Answer from the drawing. Dimensions are ordinates in mm from the lowest x, y and z of the part. Round coordinates to 2 decimals unless told otherwise and drop trailing zeros. Order: outer loops, then holes, each group sorted by start corner. A loop starts at its lowest first (then second) coordinate and runs counter-clockwise, first axis right, second up.
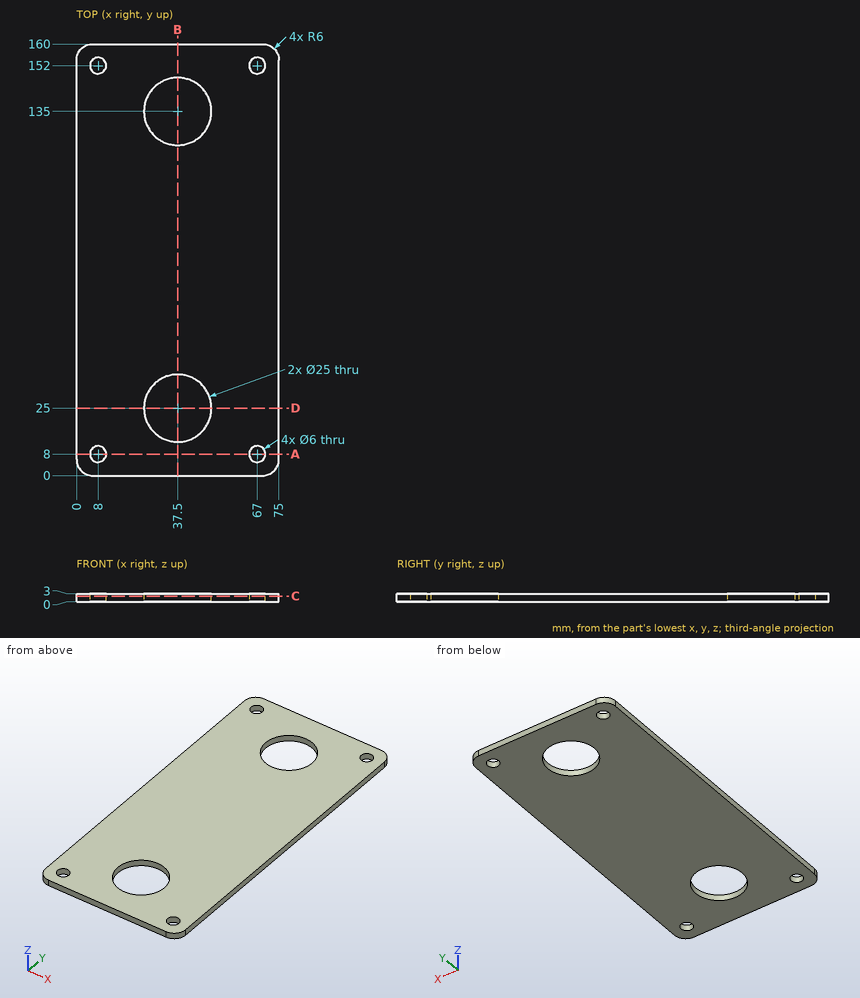
Q1. A cutting plane is placed at D-D, the plane y = 25. Give the vertices of the cut face in (x, z).
Outcome:
outline: (0, 0) - (25, 0) - (25, 3) - (0, 3) - close; (50, 0) - (75, 0) - (75, 3) - (50, 3) - close
Q2. A cutting plane is placed at C-C, the plane z = 2.05. Give the vertices of the cut face in (x, y).
Outcome:
outline: (0, 6) arc R6 ccw to (6, 0) - (69, 0) arc R6 ccw to (75, 6) - (75, 154) arc R6 ccw to (69, 160) - (6, 160) arc R6 ccw to (0, 154) - close; hole circle Ø6 at (8, 8); hole circle Ø6 at (8, 152); hole circle Ø25 at (37.5, 25); hole circle Ø25 at (37.5, 135); hole circle Ø6 at (67, 8); hole circle Ø6 at (67, 152)
Q3. A flat-ended cylindrical pin translates along its axis: pin 1 (5.5 mm diameter, centred on x = 8, y = 8, fed in from +Z). Find the tip coordinate at first contact, or state that the pin passes through.
Outcome:
pin 1: passes through
Q4. A cutting plane is placed at B-B, the plane x = 37.5. Give the vertices of the cut face in (y, z), plus the area to 3 significant figures.
Outcome:
outline: (0, 0) - (12.5, 0) - (12.5, 3) - (0, 3) - close; (37.5, 0) - (122.5, 0) - (122.5, 3) - (37.5, 3) - close; (147.5, 0) - (160, 0) - (160, 3) - (147.5, 3) - close
area: 330 mm2
Q5. Straight lines are drawn through the part: probe 1 along Y at (x, z) = (8, 1.6); probe 2 along Y at (x, z) = (37, 1.9); probe 3 along X at (y, z) = (152, 1.85). For each, find the intervals that lie inside material, in ascending order.
Outcome:
probe 1: y = 0 to 5, 11 to 149, 155 to 160
probe 2: y = 0 to 12.51, 37.49 to 122.51, 147.49 to 160
probe 3: x = 0 to 5, 11 to 64, 70 to 75
Q6. A cutting plane is placed at A-A, the plane y = 8. Give the vertices of the cut face in (x, z), plus the area to 3 significant figures.
Outcome:
outline: (0, 0) - (5, 0) - (5, 3) - (0, 3) - close; (11, 0) - (64, 0) - (64, 3) - (11, 3) - close; (70, 0) - (75, 0) - (75, 3) - (70, 3) - close
area: 189 mm2
